Read the model definition and answer for the solid it produces. Units are mm, in the model's axes. A direction names the side the tool comes from. Coordinates: 2 decimals unless noted, no trailing zeros. Order: outer loops, then holes, each group sorted by start corner. A loop starts at its lowest first (then second) coordinate and runs counter-clockwise, first axis right, second up. Notation, with made-up numbers: (70.25, -5.75) - (128.25, -5.75) arc R35 cw to (128.25, 27.25) - close; hole circle Ø11 at (35, 19.25). An arc over 180 degrees is marked (long way). Use one line per item in the form item = value. Start each with the question number.
Autodesk Inventor part; units mm, degrees
ref_plane "YZ Plane" through (0, 0, 0) normal (1, 0, 0) x (0, 1, 0)
ref_plane "XZ Plane" through (0, 0, 0) normal (0, 1, 0) x (-1, 0, 0)
ref_plane "XY Plane" through (0, 0, 0) normal (0, 0, 1) x (1, 0, 0)
sketch "Sketch1" plane through (0, 0, 0) normal (0, 1, 0) x (-1, 0, 0)
  line L0 (0, 0) -> (0, 76.2)
  line L1 (0, 0) -> (76.2, 0)
  line L2 (30.48, 27.94) -> (76.2, 27.94)
  line L3 (76.2, 27.94) -> (76.2, 18.415)
  line L4 (76.2, 0) -> (76.2, 9.525)
  line L5 (76.2, 18.415) -> (57.15, 13.97)
  line L6 (57.15, 13.97) -> (76.2, 9.525)
  line L7 (63.5, 76.2) -> (63.5, 55.88)
  line L8 (63.5, 55.88) -> (30.48, 55.88)
  line L9 (30.48, 55.88) -> (30.48, 27.94)
  line L10 (63.5, 76.2) -> (0, 76.2)
  dimension "d4" = 9.525
  dimension "d6" = 19.05
  dimension "d35" = 76.2
  dimension "d37" = 27.94
  dimension "d38" = 76.2
  dimension "d39" = 63.5
  dimension "d40" = 27.94
  dimension "d41" = 30.48
extrude "Extrusion1" add sketch "Sketch1" along normal blind 76.2
fillet "Fillet1" radius 6.35 1 edges at (-76.2, 38.1, 27.94)
fillet "Fillet2" radius 3.175 1 edges at (-57.15, 38.1, 13.97)
fillet "Fillet3" radius 3.175 1 edges at (-76.2, 38.1, 18.415)
fillet "Fillet4" radius 3.175 1 edges at (-76.2, 38.1, 9.525)
fillet "Fillet5" radius 6.35 1 edges at (-63.5, 38.1, 55.88)
fillet "Fillet6" radius 6.35 1 edges at (-30.48, 38.1, 27.94)
fillet "Fillet7" radius 6.35 1 edges at (-30.48, 38.1, 55.88)
sketch "Sketch4" plane through (-63.5, 0, 76.2) normal (0, 0, 1) x (1, 0, 0)
  line L0 (63.5, 11.43) -> (38.1, 11.43)
  line L1 (38.1, 11.43) -> (38.1, 64.77)
  line L2 (38.1, 64.77) -> (63.5, 64.77)
  line L3 (63.5, 64.77) -> (63.5, 11.43)
  line L4 (63.5, 0) -> (0, 0)
  line L5 (63.5, 76.2) -> (0, 76.2) construction
  line L6 (63.5, 0) -> (63.5, 76.2)
  dimension "d42" = 53.34
  dimension "d43" = 25.4
  dimension "d44" = 11.43
  dimension "d45" = 0
extrude "Extrusion4" cut sketch "Sketch4" against normal blind 44.45
sketch "Sketch5" plane through (0, 0, 76.2) normal (1, 0, 0) x (0, 0, -1)
  line L0 (76.2, 11.43) -> (50.8, 11.43)
  line L1 (50.8, 11.43) -> (50.8, 64.77)
  line L2 (50.8, 64.77) -> (76.2, 64.77)
  line L3 (76.2, 64.77) -> (76.2, 11.43)
  line L4 (76.2, 0) -> (76.2, 76.2)
  line L5 (0, 76.2) -> (76.2, 76.2)
  dimension "d48" = 53.34
  dimension "d49" = 25.4
  dimension "d50" = 0
  dimension "d51" = 11.43
extrude "Extrusion5" cut sketch "Sketch5" against normal blind 50.8
properties part number "Hook2"
Q1. A cutting plane is placed at A-A (x = -47). Give the vertices of the cut face in (y, z).
Q2. A cutting plane is placed at C-C (z = 71). Give the vertices of the cut face in (x, y), then the cut area to 3 significant figures.
Q3. For a pull along Z with two mould halves and no side action, classify faces 1 (the flat face through (-25, 64.77, 13)), 2 (the flat face through (-39, 38, 76.2)), 3 (the cylindrical face through (-32.29, 38.63, 29.85)), 4 (the cylindrical face through (-75.531, 38.633, 8.956)) as +Z half, -Z half, draft (parallel to the pull), parting line (faces both ways), or undercut.
Q4. Which of the six approach directions +Z, -Z, +X, -X, +Y, -Y give full straight-line access (tool end or side, diameter ignored) to faces 5 (the cylindrical face through (-61.6, 38.6, 57.7)), 6 (the flat face through (-13, 64.77, 54)), 7 (the flat face through (-63.5, 38, 69)), 8 (the flat face through (-50.8, 38, 13)), 9 (the flat face through (-29, 76.2, 39))?
Q5. A cutting plane is placed at D-D (x = -16.5). Give the vertices of the cut face in (y, z).
Q6. Given P1, Ø7.5, axis at x = -17, y = 25.5, coming from the +Z side; P2, Ø4, axis at x = -9, y = 26.5, coming from the -Z side; P3, Ø13.5, axis at y = 36.5, z = 44, coming from the +X side, each flat-ended and moving along its own axis, determine where each tip first touches the part or whether it passes through.
Q7. Consider probe 1 along Y at (x, z) = (-12, 34.5); probe 2 along Z at (x, y) = (-50, 4.5); probe 3 along X at (y, z) = (29, 50). Determine where each line is inside the solid, lowest interval first.
Result sheet:
q1.outline = (0, 0) - (11.43, 0) - (11.43, 25.4) - (64.77, 25.4) - (64.77, 0) - (76.2, 0) - (76.2, 27.94) - (0, 27.94) - close; (0, 55.88) - (76.2, 55.88) - (76.2, 76.2) - (0, 76.2) - close
q2.outline = (-63.5, 0) - (0, 0) - (0, 11.43) - (-25.4, 11.43) - (-25.4, 64.77) - (0, 64.77) - (0, 76.2) - (-63.5, 76.2) - close
q2.area = 3,480 mm^2
q3.face_1 = draft
q3.face_2 = +Z half
q3.face_3 = undercut
q3.face_4 = undercut
q4.face_5 = -X, +Y, -Y
q4.face_6 = +Z, +X
q4.face_7 = +Z, -X, +Y, -Y
q4.face_8 = -Z, +X
q4.face_9 = +Z, -Z, +X, -X, +Y
q5.outline = (0, 0) - (11.43, 0) - (11.43, 25.4) - (64.77, 25.4) - (64.77, 0) - (76.2, 0) - (76.2, 76.2) - (64.77, 76.2) - (64.77, 31.75) - (11.43, 31.75) - (11.43, 76.2) - (0, 76.2) - close
q6.P1 = 31.75
q6.P2 = 25.4
q6.P3 = -25.4
q7.probe_1 = 0 to 11.43, 64.77 to 76.2
q7.probe_2 = 0 to 27.94, 55.88 to 76.2
q7.probe_3 = -30.5 to -25.4
